Can you work these out from the model? Positions are in its coordinate system, mm. A direction names the side the tool comes from. Give positions to 0.01 mm unless a question says otherwise; leave off trailing zeros. Order: outer loops, then holes, each group sorted by start corner. A loop starts at its lowest first (then second) coordinate and runs counter-clockwise, first axis right, second up. Notation, with made-up numbers: M 60.5,60.25 L 114.5,60.25 A20 cw 114.5,94.25 Z; hole C -20,43 d7. An arc over 180 degrees is marked long. Use a Markdown table: item, result. Add a question column.
from build123d import *

# Parameters (mm, degrees)
F1_DEPTH = 12.7
F2_T     = -2.54
F4_DEPTH = 25.4


with BuildPart() as f1:
    # F0 (on Top) → F1 (new body)
    with BuildSketch(Plane.XY):
        with BuildLine():
            Line((0, -12.5342045865), (0, 12.8657954135))
            Line((0, 12.8657954135), (-165.0920747663, 12.8657954135))
            ThreePointArc((-165.0920747663, 12.8657954135), (-161.1142829028, 6.9718649096), (-159.7163041564, 0))
            ThreePointArc((-159.7163041564, 0), (-161.0258711618, -6.756378992), (-164.7649023499, -12.5342045865))
            Line((-164.7649023499, -12.5342045865), (0, -12.5342045865))
        make_face()
        with BuildLine():
            ThreePointArc((-159.7163041564, 0), (-161.1142829028, 6.9718649096), (-165.0920747663, 12.8657954135))
            Line((-165.0920747663, 12.8657954135), (-177.8, 12.8657954135))
            Line((-177.8, 12.8657954135), (-177.8, -12.5342045865))
            Line((-177.8, -12.5342045865), (-164.7649023499, -12.5342045865))
            ThreePointArc((-164.7649023499, -12.5342045865), (-161.0258711618, -6.756378992), (-159.7163041564, 0))
        make_face()
        with BuildLine():
            Line((-177.8, 12.8657954135), (-165.0920747663, 12.8657954135))
            ThreePointArc((-165.0920747663, 12.8657954135), (-195.8821958511, -0.232913217), (-164.7649023499, -12.5342045865))
            Line((-164.7649023499, -12.5342045865), (-177.8, -12.5342045865))
            Line((-177.8, -12.5342045865), (-177.8, 12.8657954135))
        make_face()
    extrude(amount=-F1_DEPTH)

    # F2
    f2_openings = [f1.faces().sort_by_distance(p)[0] for p in [
        (-100.144903, 0.13551, -12.7),
    ]]
    offset(amount=F2_T, openings=f2_openings, kind=Kind.INTERSECTION)

    # F4 (add): a face of the model
    f4_faces = [f1.faces().sort_by_distance(p)[0] for p in [
        (-100.8594782895, 0.1367235589, -2.54),
    ]]
    extrude(f4_faces, amount=F4_DEPTH)


solid = f1.part
1. If we section it at B-B, the plane z = -5.5: List the corners of the cut face in (x, y) for me.
2. If we section it at C-C, the plane x = -155: List the corners of the cut face in (y, z) for me.
3. On a 3-axis mill with a long thin cutter (end or side, diameter ignored), from which of +Z, -Z, +X, -X, +Y, -Y can I reach the whole of each face in a straight line? I mean faces 1 (the face through (-81, 12.866, -6)), 2 (the face through (-84, -12.534, -6)), 3 (the face through (-2.54, 0, -20)), 4 (the face through (-83, -9.994, -20)), 5 (the face through (-193.34, 0.31, -20.21)). Say none if no direction works.
4. I need wall thicknesses on L1, parallel to Y at x = -145, z = -14.75; L2, parallel to X at y = 1, z = -10.5; L3, parallel to Y at x = -38, z = -5. Which ranges of each line are inside material? Lowest first, please. Write a range as [from, to].
5. Will these pins go through, and if not, where does the flat tip stop? pin 1 (3 mm diameter, centred on x = -167.5, z = -4, fed in from +Y); pin 2 (10 mm diameter, centred on x = -44.5, z = -7.5, fed in from +Y); pin 3 (4.5 mm diameter, centred on y = 2.5, z = -20.5, fed in from +X).
6. If we section it at A-A, the plane x = -177.8: List the corners of the cut face in (y, z) for me, then the cut area to 3 significant figures.
7. If we section it at D-D, the plane z = -18: List the corners of the cut face in (x, y) for me, then the cut area to 3 significant figures.
Geometry results:
| question | item | result |
|---|---|---|
| 1 | outline | M -165.09,12.87 A18.08 ccw long -164.76,-12.53 L 0,-12.53 L 0,12.87 Z |
| 2 | outline | M -12.53,-12.7 L -9.99,-12.7 L -9.99,-27.94 L 10.33,-27.94 L 10.33,-12.7 L 12.87,-12.7 L 12.87,0 L -12.53,0 Z |
| 3 | face 1 | +Z, -Z, +X, +Y |
| 3 | face 2 | +Z, -Z, +X, -Y |
| 3 | face 3 | -Z, +X, +Y, -Y |
| 3 | face 4 | -Z, +X, -Y |
| 3 | face 5 | -Z |
| 4 | L1 | y = [-9.99, 10.33] |
| 4 | L2 | x = [-195.86, 0] |
| 4 | L3 | y = [-12.53, 12.87] |
| 5 | pin 1 | stops at y = 15.8 |
| 5 | pin 2 | stops at y = 12.87 |
| 5 | pin 3 | stops at x = -2.54 |
| 6 | outline | M -18.08,-12.7 L -15.54,-12.7 L -15.54,-27.94 L 15.54,-27.94 L 15.54,-12.7 L 18.08,-12.7 L 18.08,0 L -18.08,0 Z |
| 6 | area | 933 mm^2 |
| 7 | outline | M -166.18,10.33 A15.54 ccw long -165.9,-9.99 L -2.54,-9.99 L -2.54,10.33 Z |
| 7 | area | 4,030 mm^2 |
